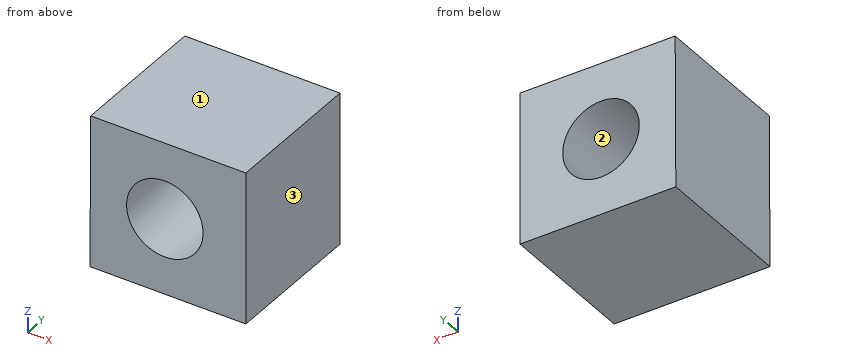
```python
from build123d import *

# Parameters (mm, degrees)
F2_DEPTH = 142.2567795962
F4_D     = 76.2


with BuildPart() as f2:
    # F1 (on face) → F2 (new body)
    with BuildSketch(Plane.XZ):
        Polygon((80.6021243334, 75.9551972151), (-73.8069862127, 75.9551972151), (-74.4586139917, -75.3483995795), (80.6021243334, -75.3483995795), align=None)
    extrude(amount=F2_DEPTH)

    # F4 (through all)
    with Locations(Plane.XZ.offset(142.2567795962)):
        with Locations((0, 0)):
            Hole(F4_D / 2)


solid = f2.part
```
Can you work these out from the model? Positions are in its coordinate system, mm. Face numbers are marked on the shaded views. Give positions to 0.01 mm unless a question says otherwise; leave off trailing zeros. Order: outer loops, then holes, each group sorted by start corner. A loop starts at its lowest first (then second) coordinate and runs counter-clockwise, first axis right, second up. Notation, with made-up numbers: (-8, 73.25) - (34, 73.25) arc R27 cw to (34, 93.25) - close; hole circle Ø7 at (-38.5, 40). An arc over 180 degrees is marked (long way). Use a Markdown table: item, result. Add a question column.
Q1. I'm going to push flat-ended pins straight in: pin 1 (1.5 mm diameter, centred on y = -55.5, z = -33.5, fed in from -X); pin 2 (3 mm diameter, centred on y = -58.5, z = -12, fed in from -X). Where does each tip first touch, or does it pass through?
Q2. If we section it at A-A on x = 0: Write out the boundary of the cut face in (y, z), plus the area to 3 significant figures.
Q3. If we section it at B-B on y = -130.5: Write out the boundary of the cut face in (x, z).
Q4. Please list where these lines run through material, in increasing order: line 1 along Z through (x, y) = (0, -84.5); line 2 along X through (y, z) = (-15, -26); line 3 along X through (y, z) = (-122, -13).
Q5. If we section it at C-C on z = 0: Write out the boundary of the cut face in (x, y), plus the area to 3 significant figures.
Q6. If we mould it in two halves opening along X, with no side actions, what happens to the marked faces 1, 2 and 3? For each: released by +X, released by -X, zero draft, split by the parting line, or undercut.
Answers follow:
| question | item | result |
|---|---|---|
| 1 | pin 1 | stops at x = -74.28 |
| 1 | pin 2 | stops at x = -74.19 |
| 2 | outline | (-142.26, -75.35) - (0, -75.35) - (0, -38.1) - (-142.26, -38.1) - close; (-142.26, 38.1) - (0, 38.1) - (0, 75.96) - (-142.26, 75.96) - close |
| 2 | area | 10,700 mm^2 |
| 3 | outline | (-74.46, -75.35) - (80.6, -75.35) - (80.6, 75.96) - (-73.81, 75.96) - close; hole circle Ø76.2 at (0, 0) |
| 4 | line 1 | z = -75.35 to -38.1, 38.1 to 75.96 |
| 4 | line 2 | x = -74.25 to -27.85, 27.85 to 80.6 |
| 4 | line 3 | x = -74.19 to -35.81, 35.81 to 80.6 |
| 5 | outline | (-74.13, -142.26) - (-38.1, -142.26) - (-38.1, 0) - (-74.13, 0) - close; (38.1, -142.26) - (80.6, -142.26) - (80.6, 0) - (38.1, 0) - close |
| 5 | area | 11,200 mm^2 |
| 6 | face 1 | zero draft |
| 6 | face 2 | undercut |
| 6 | face 3 | released by +X |
